```python
from build123d import *

# Parameters (mm, degrees)
F1_DEPTH        = 5
F4_R            = 8.05
F5_DEPTH        = 5.001
F6_R            = 5.08
F7_R            = 8.05
F8_DEPTH        = 5.001
F8_COPIES_COUNT = 4


# Not quite as in the source:
# - a pattern or mirror of a feature is missing from the dataset's text; its kind, count and spacing are read off the source's solid


with BuildPart() as f1:
    # F0 (on Front) → F1 (new body)
    with BuildSketch(Plane.XZ):
        with BuildLine():
            Line((-40, 23.4314575051), (-40, 0))
            Line((-40, 0), (0, 0))
            Line((0, 0), (0, 40))
            Line((0, 40), (-23.4314575051, 40))
            ThreePointArc((-23.4314575051, 40), (-26.5071641246, 26.5071641246), (-40, 23.4314575051))
        make_face()
    extrude(amount=F1_DEPTH)

    # F2: F1 across face


with BuildPart() as f1_1:
    add(f1.part)
    add(f1.part.mirror(Plane(origin=(0, -2.5, 20), x_dir=(0, 1, 0), z_dir=(1, 0, 0))))

    # F3: F1 across face


with BuildPart() as f1_2:
    add(f1_1.part)
    add(f1_1.part.mirror(Plane(origin=(0, -2.5, 0), x_dir=(1, 0, 0), z_dir=(0, 0, -1))))

    # F4 (on face) → F5 (cut, through all)
    with BuildSketch(Plane.XZ.offset(5)):
        Circle(F4_R)
    extrude(amount=-F5_DEPTH, mode=Mode.SUBTRACT)

    # F6
    f6_edges = [f1_2.edges().sort_by_distance(p)[0] for p in [
        (-40, -2.5, 23.431458),
        (-23.431458, -2.5, 40),
        (23.431458, -2.5, 40),
        (40, -2.5, 23.431458),
        (40, -2.5, -23.431458),
        (23.431458, -2.5, -40),
        (-40, -2.5, -23.431458),
        (-23.431458, -2.5, -40),
    ]]
    fillet(f6_edges, radius=F6_R)

    # F7 (on face) → F8 (cut, through all)
    with BuildSketch(Plane.XZ.offset(5)):
        with Locations((0, 27.7070477605)):
            Circle(F7_R)
    f8 = extrude(amount=-F8_DEPTH, mode=Mode.SUBTRACT)

    # F8_copies: F8 ×4 about axis
    f8_copies_axis = Axis((0, 0, 0), (0, 1, 0))
    for i in range(1, F8_COPIES_COUNT):
        add(f8.rotate(f8_copies_axis, i * 360 / F8_COPIES_COUNT), mode=Mode.SUBTRACT)


solid = f1_2.part
```
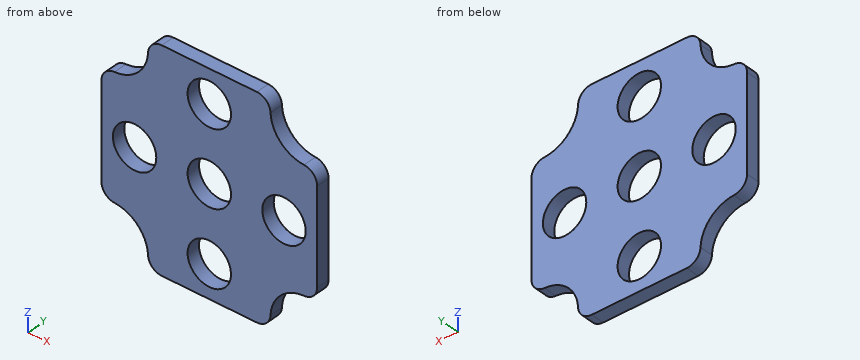
Check sheet for the modelled part. Datum: model origin and axes. Units: mm. Give positions to 0.01 mm unless a question says otherwise; leave off trailing zeros. Write each loop counter-clockwise with the first axis right and the second up, starting at its lowest first coordinate (ties: lowest second). Pieces come first, ordered by that corner, then holes. Notation, with made-up numbers: (34.5, 10) -> (39.5, 10) arc R20 ccw to (39.5, 31) -> close; hole circle Ø11 at (67.5, 76). An arc over 180 degrees is marked (long way). Use CSV: the item, a comma, the result in double quotes. Start each with the question number.
Q1. Cross-section at B-B on x = -34. Enter the section's corners in (y, z), and give its area (3 significant figures).
Q2. Depth check by flat-ended pin: P1, Ø3, axis at y = -1.5, z = -21, coming from the +X side; P2, Ø18.5, axis at x = 0, z = 0, coming from the -Y side. Enter the tip coordinate at first touch or a pass-through.
Q3. Cross-section at D-D on y = -4.1. Enter the section's corners in (x, z), and give its area (3 significant figures).
Q4. Scan lines: line 1 along Z through (x, y) = (0, -2.85); line 2 along X through (y, z) = (-4.5, -4); line 3 along Z through (x, y) = (-22, -0.9). Record each from-to range of solid material in increasing order.
Q5. Cross-section at C-C on x = 0. Enter the section's corners in (y, z).
Q6. Cross-section at A-A on z = 0. Enter the section's corners in (x, y).
Working result:
1,outline,"(-5, -22.81) -> (0, -22.81) -> (0, -5.02) -> (-5, -5.02) -> close; (-5, 5.02) -> (0, 5.02) -> (0, 22.81) -> (-5, 22.81) -> close"
1,area,"178 mm^2"
2,P1,"stops at x = 39.65"
2,P2,"stops at y = -5"
3,outline,"(-40, -17.64) arc R5.08 ccw to (-35.14, -22.71) arc R13 cw to (-22.71, -35.14) arc R5.08 ccw to (-17.64, -40) -> (17.64, -40) arc R5.08 ccw to (22.71, -35.14) arc R13 cw to (35.14, -22.71) arc R5.08 ccw to (40, -17.64) -> (40, 17.64) arc R5.08 ccw to (35.14, 22.71) arc R13 cw to (22.71, 35.14) arc R5.08 ccw to (17.64, 40) -> (-17.64, 40) arc R5.08 ccw to (-22.71, 35.14) arc R13 cw to (-35.14, 22.71) arc R5.08 ccw to (-40, 17.64) -> close; hole circle Ø16.1 at (-27.71, 0); hole circle Ø16.1 at (0, -27.71); hole circle Ø16.1 at (0, 0); hole circle Ø16.1 at (0, 27.71); hole circle Ø16.1 at (27.71, 0)"
3,area,"4,290 mm^2"
4,line 1,"z = -40 to -35.76, -19.66 to -8.05, 8.05 to 19.66, 35.76 to 40"
4,line 2,"x = -40 to -34.69, -20.72 to -6.99, 6.99 to 20.72, 34.69 to 40"
4,line 3,"z = -37.52 to -5.68, 5.68 to 37.52"
5,outline,"(-5, -40) -> (0, -40) -> (0, -35.76) -> (-5, -35.76) -> close; (-5, -19.66) -> (0, -19.66) -> (0, -8.05) -> (-5, -8.05) -> close; (-5, 8.05) -> (0, 8.05) -> (0, 19.66) -> (-5, 19.66) -> close; (-5, 35.76) -> (0, 35.76) -> (0, 40) -> (-5, 40) -> close"
6,outline,"(-40, -5) -> (-35.76, -5) -> (-35.76, 0) -> (-40, 0) -> close; (-19.66, -5) -> (-8.05, -5) -> (-8.05, 0) -> (-19.66, 0) -> close; (8.05, -5) -> (19.66, -5) -> (19.66, 0) -> (8.05, 0) -> close; (35.76, -5) -> (40, -5) -> (40, 0) -> (35.76, 0) -> close"
